Can you work these out from the model? Positions are in its coordinate system, mm. Give positions to 0.01 mm unless a question says otherwise; leave off trailing zeros. Order: outer loops, then holes, each group sorted by start corner. A loop starts at its lowest first (then second) coordinate and runs counter-clockwise, first axis right, second up. Notation, with made-up numbers: M 9,25 L 59,25 A21 ccw 59,31 Z; hole C 84,54.25 d6. An arc over 180 degrees is marked long. Answer as a JSON object with one key per item and string values.
```python
from build123d import *

# Parameters (mm, degrees)
SKETCH1_R                       = 40
SKETCH1_R_2                     = 30
BOSS_EXTRUDE1_DEPTH             = 8
M4X0_7_TAPPED_HOLE1_D           = 3.3
M4X0_7_TAPPED_HOLE1_CSINK_D     = 4.05
M4X0_7_TAPPED_HOLE1_CSINK_ANGLE = 90
CIRPATTERN1_COUNT               = 12


with BuildPart() as part:
    # Sketch1 → Boss-Extrude1 (new body)
    with BuildSketch(Plane.XY):
        Circle(SKETCH1_R)
        Circle(SKETCH1_R_2, mode=Mode.SUBTRACT)
    extrude(amount=-BOSS_EXTRUDE1_DEPTH)

    # M4x0.7 Tapped Hole1 (through all)
    with Locations(Plane.XY):
        with Locations((0, 36.25)):
            m4x0_7_tapped_hole1 = CounterSinkHole(M4X0_7_TAPPED_HOLE1_D / 2, M4X0_7_TAPPED_HOLE1_CSINK_D / 2, counter_sink_angle=M4X0_7_TAPPED_HOLE1_CSINK_ANGLE)

    # CirPattern1: M4x0.7 Tapped Hole1 ×12 about axis
    cirpattern1_axis = Axis((0, 0, 0), (0, 0, 1))
    for i in range(1, CIRPATTERN1_COUNT):
        add(m4x0_7_tapped_hole1.rotate(cirpattern1_axis, i * 360 / CIRPATTERN1_COUNT), mode=Mode.SUBTRACT)


solid = part.part
```
1) I need wall thicknesses on L1, parallel to Y at x = -17.5, z = -0.25; L2, parallel to X at y = 32, z = -6.5; L3, parallel to Y at x = 30.5, z = -7.5. Which ranges of each line are inside material? Lowest first, please.
Results found:
{"L1": "y = -35.97 to -33.05, -29.73 to -24.37, 24.37 to 29.73, 33.05 to 35.97", "L2": "x = -24 to -19.66, -16.59 to 16.59, 19.66 to 24", "L3": "y = -25.88 to -19.51, -16.74 to 16.74, 19.51 to 25.88"}
2) I want a section at A-A on y = -24.5. Write out the boundary of the cut face in (x, z).
Results found:
{"outline": "M -31.62,-8 L -17.31,-8 L -17.31,0 L -31.62,0 Z; M 17.31,-8 L 31.62,-8 L 31.62,0 L 17.31,0 Z"}
3) I'm going to push flat-ended pins straight in: pin 1 Ø4 at (x, y) = (36.25, 0) entering from +Z (3 decimals); pin 2 Ø3 at (x, y) = (31.39, 18.13) entering from -Z; pin 3 Ø4 at (y, z) = (-2.5, -6.5) entering from +X; pin 4 Ø4.5 at (x, y) = (0, -36.25) entering from -Z. Where does each tip first touch, or does it pass through?
Results found:
{"pin 1": "stops at z = -0.025", "pin 2": "passes through", "pin 3": "stops at x = 40", "pin 4": "stops at z = -8"}
4) I want a section at B-B on x = 36.25. Write out the boundary of the cut face in (y, z) (3 decimals).
Results found:
{"outline": "M -16.91,-8 L -1.65,-8 L -1.65,-0.375 L -2.025,0 L -16.91,0 Z; M 1.65,-8 L 16.91,-8 L 16.91,0 L 2.025,0 L 1.65,-0.375 Z"}
5) Thinking about a two-plate mould opening in Y: for faces 1 (the face through (26.5, 15, -8)), 2 (the face through (-8.67, -39.05, -3.94)), 3 (the face through (-29.87, 18.76, -4.24)), which applies, pulls with the +Y half, pulls with the -Y half, needs draft (parallel to the pull), parting line crosses it, or undercut?
Results found:
{"face 1": "needs draft", "face 2": "parting line crosses it", "face 3": "undercut"}
6) I want a section at C-C on z = -2.25. Count the separate pieces of the cut face and the enclosed holes in it, and give its area (3 significant figures).
Results found:
{"separate pieces": "1", "enclosed holes": "13", "area": "2,100 mm²"}
7) I want a section at D-D on y = -9. Write out the boundary of the cut face in (x, z), and give its area (3 significant figures).
Results found:
{"outline": "M -38.97,-8 L -28.62,-8 L -28.62,0 L -38.97,0 Z; M 28.62,-8 L 38.97,-8 L 38.97,0 L 28.62,0 Z", "area": "166 mm²"}
